Input: part model. Units: mm. Frame: model coordinates. A direction names the side the tool comes from. Coordinates: 2 decimals unless noted, no trailing zeros. Write each loop counter-clockwise with the first axis right and the second up, starting at its lowest first coordinate (ties: lowest second). Pieces come first, ordered by that corner, then holes. Notation, with made-up numbers: M 59,-34 L 92,-34 A15 cw 92,-5 Z; hole C -15.75,68 d8. An arc over 180 degrees is marked long. Use one line per item in the form item = value.
from build123d import *

# Parameters (mm, degrees)
SKETCH1_R           = 63
SKETCH1_R_2         = 2.625
BOSS_EXTRUDE1_DEPTH = 7
SKETCH2_R           = 4.375
CUT_EXTRUDE1_DEPTH  = 5
CUT_EXTRUDE2_REACH  = 91.37
SKETCH3_W           = 40
SKETCH3_H           = 50


with BuildPart() as part:
    # Sketch1 → Boss-Extrude1 (new body)
    with BuildSketch(Plane(origin=(0, 0, 0), x_dir=(1, 0, 0), z_dir=(0, 1, 0))):
        with Locations(Location((0, 0, 0), (0, 0, 270))):
            Circle(SKETCH1_R)
        with Locations(Location((-40, 15, 0), (0, 0, 270))):
            Circle(SKETCH1_R_2, mode=Mode.SUBTRACT)
        with Locations(Location((-40, -15, 0), (0, 0, 270))):
            Circle(SKETCH1_R_2, mode=Mode.SUBTRACT)
        with Locations(Location((40, 15, 0), (0, 0, 270))):
            Circle(SKETCH1_R_2, mode=Mode.SUBTRACT)
        with Locations(Location((40, -15, 0), (0, 0, 270))):
            Circle(SKETCH1_R_2, mode=Mode.SUBTRACT)
    extrude(amount=BOSS_EXTRUDE1_DEPTH)

    # Sketch2 → Cut-Extrude1 (cut)
    with BuildSketch(Plane(origin=(0, 7, 0), x_dir=(1, 0, 0), z_dir=(0, 1, 0))):
        with Locations(Location((-40, 15, 0), (0, 0, 270))):
            Circle(SKETCH2_R)
        with Locations(Location((-40, -15, 0), (0, 0, 270))):
            Circle(SKETCH2_R)
        with Locations(Location((40, 15, 0), (0, 0, 270))):
            Circle(SKETCH2_R)
        with Locations(Location((40, -15, 0), (0, 0, 270))):
            Circle(SKETCH2_R)
    extrude(amount=-CUT_EXTRUDE1_DEPTH, mode=Mode.SUBTRACT)

    # Chamfer1: read off the stored shape, not the designer's step
    # Chamfer1 outline → Chamfer1 (revolve, cut)
    with BuildSketch(Plane.XY):
        Polygon((63, 7), (60, 7), (63, 4), align=None)
    revolve(axis=Axis((0, 0, 0), (0, 1, 0)), mode=Mode.SUBTRACT)

    # Cut-Extrude2: up to this face of the body (flat: up to its plane)
    cut_extrude2_end = Plane(part.part.faces().sort_by_distance((0, 0, 0))[0])
    # Sketch3 → Cut-Extrude2 (cut, up to the picked face)
    with BuildSketch(Plane(origin=(0, 7, 0), x_dir=(1, 0, 0), z_dir=(0, 1, 0)), mode=Mode.PRIVATE) as cut_extrude2_sk1:
        with Locations((0, 40)):
            Rectangle(SKETCH3_W, SKETCH3_H)
    cut_extrude2_tool1 = split(extrude(cut_extrude2_sk1.sketch, amount=-CUT_EXTRUDE2_REACH, mode=Mode.PRIVATE), bisect_by=cut_extrude2_end, keep=Keep.BOTH, mode=Mode.PRIVATE)
    add(cut_extrude2_tool1.solids().sort_by(Axis((0, 7, -40), (0, -1, 0)))[0], mode=Mode.SUBTRACT)


solid = part.part
(1) Pull-direction query (X, two-part tool) for faces 1 (the flat face through (1, 7, 1)), 2 (the cylindrical face through (44.338, 4.535, -15.57)), 3 (the conical face through (-2.374, 6.812, 60.141)); classes: pulls with the +X half, pulls with the -X half, needs draft (parallel to the pull), parting line crosses it, or undercut.
Computed:
face_1 = needs draft
face_2 = undercut
face_3 = parting line crosses it
(2) Line query: probe 1 along X at (y, z) = (5.75, -18.5) (3 decimals); probe 2 along Z at (x, y) = (-40, 1.3) (3 decimals); probe 3 along Z at (x, y) = (44, 4.5). Output: solid intervals per line, ascending.
Computed:
probe_1 = -58.389 to -42.625, -37.375 to -20, 20 to 37.375, 42.625 to 58.389
probe_2 = -48.672 to -17.625, -12.375 to 12.375, 17.625 to 48.672
probe_3 = -44.39 to -16.77, -13.23 to 13.23, 16.77 to 44.39
(3) First-contact query: pin 1 Ø7 at (x, z) = (40, 15) entering from +Y; pin 2 Ø1 at (x, y) = (-41.5, 3.5) entering from -Z; pin 3 Ø4 at (x, y) = (-15, 4.5) entering from -Z; pin 4 Ø3 at (x, z) = (-40, -15) entering from -Y (3 decimals). Flat tips, straight axial feed; report the tip coordinate or a pass-through.
Computed:
pin_1 = 2
pin_2 = -47.83
pin_3 = -15
pin_4 = through
(4) Section query D-D on x = 0. Return the cut outline in (y, z).
Computed:
outline = M 0,-15 L 7,-15 L 7,60 L 4,63 L 0,63 Z
(5) Set-up query: faces 4 (the cylindrical face through (-39.885, 0.986, -17.622)), 5 (the cylindrical face through (44.338, 4.535, 14.43)), 6 (the flat face through (-20, 4, -37)). Return all of +Z, -Z, +X, -X, +Y, -Y with unobstructed straight access to the full face (end or side cutting, diameter ignored); none if empty.
Computed:
face_4 = +Y, -Y
face_5 = +Y
face_6 = -Z, +Y, -Y
(6) Section query A-A on y = 5.75. Return the cut outline in (x, z) (3 decimals).
Computed:
outline = M -20,-57.893 L -20,-15 L 20,-15 L 20,-57.893 A61.25 ccw long Z; hole C -40,-15 d8.75; hole C -40,15 d8.75; hole C 40,-15 d8.75; hole C 40,15 d8.75
(7) Section query B-B on x = -40. State how many separate pieces and enclosed holes the cut face has, plus the area to 3 significant figures.
Computed:
separate_pieces = 3
enclosed_holes = 0
area = 561 mm^2
